For this review, take the finished solid that the model builds, in its own axes (mm). A direction names the side the tool comes from. Round coordinates to 2 decimals unless told otherwise and drop trailing zeros. Loops run counter-clockwise (first coordinate to the right, second up) from the corner with the lowest first, then second, coordinate; pieces in that order, holes last.
1. Consider section A-A on z = 48. State the section outline as (x, y) points.
2. Consider section B-B on x = 0. State how many separate pieces and enclosed holes the cut face has, then the cut area to 3 significant figures.
3. Clearance check with flat-ended pins moving along their axes: pin 1 Ø9 at (x, z) = (0, -48) entering from +Y; pin 2 Ø15.5 at (x, z) = (36.434, 31.25) entering from -Y; pin 3 Ø1 at (x, y) = (-5.5, -13) entering from +Z (3 decimals); pin 4 Ø5 at (x, z) = (0, 48) entering from +Y. State where each tip first meets the part, or that it passes through.
4. Tool access review of faces 5 (the conical face through (13.19, -25.79, 9.53)), 6 (the flat face through (-5, -26.5, -17)), 7 (the cylindrical face through (12, -4, 9)): name each direction out of +Z, -Z, +X, -X, +Y, -Y from which nothing blocks a thin tool from reaching the whole face with its end or side.
5. Draft analysis for pull direction X (two halves, no side actions). For faces 1 (the conical face through (-5.097, 16.891, 22.955)), 2 (the cylindrical face through (-4.036, 7.007, -30.736)), 3 (the conical face through (13.14, -25.79, -9.6)), 4 (the flat face through (23, 6.5, 14)), state which applies: released by +X, released by -X, zero draft, split by the parting line, or undercut.
6. To check wall thickness, follow line 1 along Z through (x, y) = (0, 17.75); line 2 along Z through (x, y) = (0, 15); line 3 along X through (y, z) = (20, -31). State the ranges of each line that lie inside material, in increasing order.
Autodesk Inventor part; units mm, degrees
ref_plane "YZ Plane" through (0, 0, 0) normal (1, 0, 0) x (0, 1, 0)
ref_plane "XZ Plane" through (0, 0, 0) normal (0, 1, 0) x (-1, 0, 0)
ref_plane "XY Plane" through (0, 0, 0) normal (0, 0, 1) x (1, 0, 0)
sketch "Эскиз1" plane through (0, 0, 0) normal (0, 0, 1) x (1, 0, 0)
  line L0 (0, 26.5) -> (0, -26.5)
  line L1 (17.5, -26.5) -> (22.9019, -26.5)
  line L2 (25.5, -22) -> (25.5, 5.5)
  line L3 (17.5, -26.5) -> (17.5, 16)
  line L4 (25.5, -22) -> (22.9019, -26.5)
  line L5 (26.5, 6.5) -> (31, 6.5)
  arc A0 (26.5, 6.5) -> (25.5, 5.5) centre (26.5, 5.5) ccw
  line L6 (31, 6.5) -> (31, 7.5)
  line L7 (31, 7.5) -> (29.5, 8.366)
  line L8 (29.5, 8.366) -> (29.5, 11)
  line L9 (31.5, 13) -> (60, 13)
  arc A1 (31.5, 13) -> (29.5, 11) centre (31.5, 11) ccw
  line L10 (60, 13) -> (60, 22.5)
  line L11 (60, 22.5) -> (38, 22.5)
  line L12 (38, 22.5) -> (36.5, 21.634)
  arc A2 (35, 22.5) -> (36.5, 21.634) centre (36, 22.5) ccw
  line L13 (35, 22.5) -> (35, 26)
  line L14 (34.7113, 26.5) -> (29.0622, 26.5)
  line L15 (29.0622, 26.5) -> (23.1443, 16.25)
  line L16 (22.7113, 16) -> (17.5, 16)
  arc A3 (22.7113, 16) -> (23.1443, 16.25) centre (22.7113, 16.5) ccw
  line L17 (35, 26) -> (34.7113, 26.5)
  point P0 (0, 0)
  point P1 (0, 0)
  point P2 (25.5, -26.5)
  point P3 (25.5, 6.5)
  point P4 (35, 26.5)
  point P5 (23, 16)
  dimension "d0" = 53
  dimension "d1" = 35
  dimension "d2" = 51
  dimension "d3" = 4.5
  dimension "d4" = 30
  dimension "d5" = 1
  dimension "d7" = 33
  dimension "d8" = 1
  dimension "d9" = 30
  dimension "d10" = 2
  dimension "d11" = 59
  dimension "d12" = 62
  dimension "d13" = 9.5
  dimension "d14" = 30
  dimension "d15" = 1
  dimension "d16" = 120
  dimension "d17" = 70
  dimension "d18" = 4
  dimension "d19" = 30
  dimension "d20" = 10.5
  dimension "d21" = 0.5
  dimension "d22" = 46
  dimension "d23" = 0.5
  dimension "d24" = 30
revolve "Вращение1" add sketch "Эскиз1" angle 360 about axis through (0, 26.5, 0) along (0, -1, 0)
sketch "Эскиз2" plane through (0, 22.5, 0) normal (0, 1, 0) x (1, 0, 0)
  circle A0 centre (0, 0) radius 48 construction
  circle A1 centre (-36.434, 31.25) radius 6
  line L0 (-36.434, 31.25) -> (-36.434, -31.25) construction
  circle A2 centre (-36.434, -31.25) radius 6
  circle A3 centre (36.434, 31.25) radius 6
  circle A4 centre (36.434, -31.25) radius 6
  circle A5 centre (0, -48) radius 4
  circle A6 centre (0, 48) radius 4
  dimension "d26" = 96
  dimension "d27" = 12
  dimension "d28" = 62.5
  dimension "d29" = 8
extrude "Выдавливание1" cut sketch "Эскиз2" against normal through all
thread "Резьба1"
thread "Резьба2"
thread "Резьба3"
thread "Резьба4"
thread "Резьба5"
thread "Резьба6"
sketch "Эскиз3" plane through (0, 16, 0) normal (0, 1, 0) x (1, 0, 0)
  circle A0 centre (0, 0) radius 15
  circle A1 centre (0, 0) radius 17.5
  circle A2 centre (0, 0) radius 17.5 construction
  line L0 (-2.5, -17.3205) -> (2.5, -17.3205) construction
  line L1 (8.1582, -15.482) -> (12.2033, -12.5431) construction
  line L2 (15.7002, -7.73) -> (17.2453, -2.9747) construction
  line L3 (17.2453, 2.9747) -> (15.7002, 7.73) construction
  line L4 (12.2033, 12.5431) -> (8.1582, 15.482) construction
  line L5 (2.5, 17.3205) -> (-2.5, 17.3205) construction
  line L6 (-8.1582, 15.482) -> (-12.2033, 12.5431) construction
  line L7 (-15.7002, 7.73) -> (-17.2453, 2.9747) construction
  line L8 (-17.2453, -2.9747) -> (-15.7002, -7.73) construction
  line L9 (-12.2033, -12.5431) -> (-8.1582, -15.482) construction
  line L10 (-2.5, -17.3205) -> (-2.9612, -14.7048)
  line L11 (-8.1582, -15.482) -> (-6.2476, -13.637)
  line L12 (2.5, -17.3205) -> (2.9612, -14.7048)
  line L13 (8.1582, -15.482) -> (6.2476, -13.637)
  line L14 (12.2033, -12.5431) -> (11.0389, -10.1559)
  line L15 (15.7002, -7.73) -> (13.07, -7.3603)
  line L16 (17.2453, -2.9747) -> (14.9002, -1.7277)
  line L17 (17.2453, 2.9747) -> (14.9002, 1.7277)
  line L18 (15.7002, 7.73) -> (13.07, 7.3603)
  line L19 (12.2033, 12.5431) -> (11.0389, 10.1559)
  line L20 (8.1582, 15.482) -> (6.2476, 13.637)
  line L21 (2.5, 17.3205) -> (2.9612, 14.7048)
  line L22 (-2.5, 17.3205) -> (-2.9612, 14.7048)
  line L23 (-8.1582, 15.482) -> (-6.2476, 13.637)
  line L24 (-12.2033, 12.5431) -> (-11.0389, 10.1559)
  line L25 (-15.7002, 7.73) -> (-13.07, 7.3603)
  line L26 (-17.2453, 2.9747) -> (-14.9002, 1.7277)
  line L27 (-17.2453, -2.9747) -> (-14.9002, -1.7277)
  line L28 (-15.7002, -7.73) -> (-13.07, -7.3603)
  line L29 (-12.2033, -12.5431) -> (-11.0389, -10.1559)
  point P0 (0, -17.3205)
  point P1 (10.1807, -14.0126)
  point P2 (16.4728, -5.3523)
  point P3 (16.4728, 5.3523)
  point P4 (10.1807, 14.0126)
  point P5 (0, 17.3205)
  point P6 (-10.1807, 14.0126)
  point P7 (-16.4728, 5.3523)
  point P8 (-16.4728, -5.3523)
  point P9 (-10.1807, -14.0126)
  point P10 (8.1582, -15.482)
  point P11 (6.2476, -13.637)
  point P12 (2.9612, -14.7048)
  point P13 (15.7002, -7.73)
  point P14 (13.07, -7.3603)
  point P15 (11.0389, -10.1559)
  point P16 (12.2033, -12.5431)
  point P17 (17.2453, 2.9747)
  point P18 (14.9002, 1.7277)
  point P19 (14.9002, -1.7277)
  point P20 (17.2453, -2.9747)
  point P21 (12.2033, 12.5431)
  point P22 (11.0389, 10.1559)
  point P23 (13.07, 7.3603)
  point P24 (15.7002, 7.73)
  point P25 (6.2476, 13.637)
  point P26 (8.1582, 15.482)
  point P27 (-6.2476, 13.637)
  point P28 (-2.9612, 14.7048)
  point P29 (-15.7002, 7.73)
  point P30 (-13.07, 7.3603)
  point P31 (-11.0389, 10.1559)
  point P32 (-12.2033, 12.5431)
  point P33 (-17.2453, -2.9747)
  point P34 (-14.9002, -1.7277)
  point P35 (-14.9002, 1.7277)
  point P36 (-17.2453, 2.9747)
  point P37 (-12.2033, -12.5431)
  point P38 (-11.0389, -10.1559)
  point P39 (-13.07, -7.3603)
  point P40 (-15.7002, -7.73)
  dimension "d44" = 30
  dimension "d45" = 5
  dimension "d48" = 360
  dimension "d50" = 100
  dimension "d51" = 56
  dimension "d54" = 360
extrude "Выдавливание2" add sketch "Эскиз3" against normal up to surface (42.5 mm away) contours A0 L17 A1 L16 | A0 L19 A1 L18 | L15 A1 L14 A0 | A0 L21 A1 L20 | L13 A1 L12 A0 | A0 L23 A1 L22 | L10 A1 L11 A0 | A0 L25 A1 L24 | L29 A1 L28 A0 | A0 L27 A1 L26
fillet "Сопряжение1" radius 0.3 20 edges at (-2.5, -5.25, -17.3205) (-8.1582, -5.25, -15.482) (2.5, -5.25, -17.3205) (8.1582, -5.25, -15.482) (15.7002, -5.25, -7.73) (12.2033, -5.25, -12.5431) (17.2453, -5.25, -2.9747) (17.2453, -5.25, 2.9747) (15.7002, -5.25, 7.73) (12.2033, -5.25, 12.5431) (8.1582, -5.25, 15.482) (2.5, -5.25, 17.3205) (-2.5, -5.25, 17.3205) (-8.1582, -5.25, 15.482) (-12.2033, -5.25, 12.5431) (-15.7002, -5.25, 7.73) (-17.2453, -5.25, 2.9747) (-17.2453, -5.25, -2.9747) (-15.7002, -5.25, -7.73) (-12.2033, -5.25, -12.5431)
sketch "Эскиз4" plane through (0, -26.5, 0) normal (0, -1, 0) x (1, 0, 0)
  circle A0 centre (0, 0) radius 17.5 construction
  arc A1 (17.2065, 3.1917) -> (15.7964, 7.5316) centre (0, 0) ccw construction
sketch "Эскиз5" plane through (0, 0, 0) normal (0, 0, 1) x (1, 0, 0)
  line L0 (-17.5, -26.5) -> (17.5, -26.5) construction
  line L1 (15, -26.5) -> (15, 16)
  line L2 (17.5, -26.5) -> (15, -25.0566)
  line L3 (-22.9019, -26.5) -> (22.9019, -26.5)
  line L4 (0, -37.1) -> (0, 37.1)
  point P0 (0, 0)
  dimension "d59" = 30
revolve "Вращение2" cut sketch "Эскиз5" angle 360 about axis through (0, -10, 0) along (0, 1, 0)
properties part number "65. Муфта вторичного вала"
Resolved:
1. outline: (-36, 13) - (-4, 13) - (-4, 22.5) - (-36, 22.5) - close; (4, 13) - (36, 13) - (36, 22.5) - (4, 22.5) - close
2. separate pieces: 4
2. enclosed holes: 0
2. area: 1,290 mm2
3. pin 1: stops at y = 22.5
3. pin 2: stops at y = 13
3. pin 3: stops at z = 25.005
3. pin 4: passes through
4. face 5: -Y
4. face 6: +Z, -Z, +X, -X, -Y
4. face 7: +Y, -Y
5. face 1: undercut
5. face 2: split by the parting line
5. face 3: undercut
5. face 4: zero draft
6. line 1: z = -60 to -52, -44 to -24.01, 24.01 to 44, 52 to 60
6. line 2: z = -60 to -52, -44 to -17.5, 17.5 to 44, 52 to 60
6. line 3: x = -51.37 to -42.43, -30.44 to 30.44, 42.43 to 51.37
